Can you work these out from the model? Positions are in its coordinate system, mm. A direction names the side the tool comes from. Give positions to 0.01 mm unless a question says otherwise; leave off trailing zeros. Loops run counter-clockwise (first coordinate to the right, second up) from the corner with the lowest first, then second, coordinate; pieces in that order, holes last. Notation, with made-up numbers: M 39,-12 L 92,-12 A10 cw 92,7 Z; hole C 73,52 d4. An arc over 180 degrees is marked long. Answer as a JSON object with one key per item and string values.
```python
from build123d import *

# Parameters (mm, degrees)
DODANIE_WYCI_GNI_CIE1_DEPTH = 15
DODANIE_WYCI_GNI_CIE2_DEPTH = 2.5
SZKIC4_R                    = 2.2
WYTNIJ_WYCI_GNI_CIE1_DEPTH  = 10
SZKIC5_R                    = 2.2
WYTNIJ_WYCI_GNI_CIE2_DEPTH  = 10
SZKIC6_R                    = 3.5
WYTNIJ_WYCI_GNI_CIE3_DEPTH  = 1


with BuildPart() as part:
    # Szkic2 → Dodanie-wyciągnięcie1 (new body)
    with BuildSketch(Plane.XY):
        Polygon((-4.489744218, 18.257150965), (-12.375242327, -9.242849035), (1.624757673, -9.242849035), (1.624757673, -6.242849035), (-8.515006169, -6.242849035), (-0.890760007, 20.346057156), (-18.08175759, 25.27549639), (-18.908669657, 22.391711302), align=None)
    extrude(amount=DODANIE_WYCI_GNI_CIE1_DEPTH)

    # Szkic3 → Dodanie-wyciągnięcie2 (add)
    with BuildSketch(Plane(origin=(0, 0, 0), x_dir=(-1, 0, 0), z_dir=(0, 0, -1))):
        Polygon((0.890760007, 20.346057156), (-1.624757673, -6.242849035), (8.515006169, -6.242849035), align=None)
    extrude(amount=-DODANIE_WYCI_GNI_CIE2_DEPTH)

    # Szkic4 → Wytnij-wyciągnięcie1 (cut)
    with BuildSketch(Plane(origin=(0, -6.242849035, 0), x_dir=(1, 0, 0), z_dir=(0, 1, 0))):
        with Locations(Location((-2.675242327, -8.75, 0), (0, 0, 180))):
            Circle(SZKIC4_R)
    extrude(amount=-WYTNIJ_WYCI_GNI_CIE1_DEPTH, mode=Mode.SUBTRACT)

    # Szkic5 → Wytnij-wyciągnięcie2 (cut)
    with BuildSketch(Plane(origin=(-6.213967486, 1.781826504, 0), x_dir=(0, 0, -1), z_dir=(0.9612616959383198, -0.27563735581699605, 0))):
        with Locations(Location((-8.75, -3.348065436, 0), (0, 0, 90))):
            Circle(SZKIC5_R)
    extrude(amount=-WYTNIJ_WYCI_GNI_CIE2_DEPTH, mode=Mode.SUBTRACT)

    # Szkic6 → Wytnij-wyciągnięcie3 (cut)
    with BuildSketch(Plane(origin=(-6.213967486, 1.781826504, 0), x_dir=(0, 0, -1), z_dir=(0.9612616959383198, -0.27563735581699605, 0))):
        with Locations(Location((-8.75, -3.348065436, 0), (0, 0, 90))):
            Circle(SZKIC6_R)
    extrude(amount=-WYTNIJ_WYCI_GNI_CIE3_DEPTH, mode=Mode.SUBTRACT)


solid = part.part
```
1) For faces 1 (the flat face through (-4.756, 6.865, 8.662)), 2 (the flat face through (-8.377, 4.7, 7.395)), 3 (the flat face through (-9.366, 22.776, 7.395)), 4 (the cylindrical face through (-4.774, -7.722, 9.411)), which set-ups out of +Z, -Z, +X, -X, +Y, -Y let a thin tool reach every point of the face, with its end or its side?
Answer list:
{"face 1": "+Z, +X", "face 2": "+Z, -Z, -X", "face 3": "+Z, -Z, +X, +Y", "face 4": "-Y"}
2) Suppose I cut it at C-C, the plane y = 14.5. Write out the boundary of the cut face in (x, z), and give its area (3 significant figures).
Answer list:
{"outline": "M -5.57,0 L -0.34,0 L -0.34,2.5 L -2.57,2.5 L -2.57,15 L -5.57,15 Z", "area": "50.6 mm^2"}
3) If we mould it in two halves opening along Z, with no side actions, what happens to faces 5 (the flat face through (-6, 8, 15)), 6 (the flat face through (1.625, -8, 7)), 7 (the flat face through (-7.897, -0.46, 6.466))? For each: +Z half, -Z half, draft (parallel to the pull), parting line (faces both ways), or undercut.
Answer list:
{"face 5": "+Z half", "face 6": "draft", "face 7": "undercut"}
4) Suppose I cut it at B-B, the plane z = 13.5. Write out the boundary of the cut face in (x, y) (1 decimal), and give its area (3 significant figures).
Answer list:
{"outline": "M -18.9,22.4 L -4.5,18.3 L -12.4,-9.2 L 1.6,-9.2 L 1.6,-6.2 L -8.5,-6.2 L -0.9,20.3 L -18.1,25.3 Z", "area": "167 mm^2"}
5) Suppose I cut it at A-A, the plane z = 8.75. Write out the boundary of the cut face in (x, y) (1 decimal).
Answer list:
{"outline": "M -18.9,22.4 L -4.5,18.3 L -9.3,1.5 L -7.5,1 L -7.1,2.2 L -6.2,1.9 L -0.9,20.3 L -18.1,25.3 Z; M -12.4,-9.2 L -4.9,-9.2 L -4.9,-6.2 L -8.5,-6.2 L -8.1,-4.8 L -9.1,-4.5 L -8.7,-3.3 L -10.5,-2.8 Z; M -0.5,-9.2 L 1.6,-9.2 L 1.6,-6.2 L -0.5,-6.2 Z"}
6) Will these pins go through, and if not, where does the flat tip stop? pin 1 Ø5 at (x, z) = (-2, 10) entering from +Y; pin 2 Ø5 at (y, z) = (19.5, 5.5) entering from +X; pin 3 Ø1 at (x, z) = (-12.5, 10) entering from -Y; pin 4 Ø6 at (y, z) = (15.5, 12) entering from +X.
Answer list:
{"pin 1": "y = 21.38", "pin 2": "x = -0.89", "pin 3": "y = -9.24", "pin 4": "x = -1.42"}
7) Please list where these lines run through material, in increasing order: line 1 along Z through (x, y) = (-1.25, -6); line 2 along Y through (x, z) = (-18, 6.25); line 3 along X through (y, z) = (17, 8.25). Write a range as from..to.
Answer list:
{"line 1": "0..2.5", "line 2": "22.13..25.25", "line 3": "-4.85..-1.85"}
8) Suppose I cut it at D-D, the plane x = -14.5. Write out the boundary of the cut face in (y, z).
Answer list:
{"outline": "M 21.13,0 L 24.25,0 L 24.25,15 L 21.13,15 Z"}
